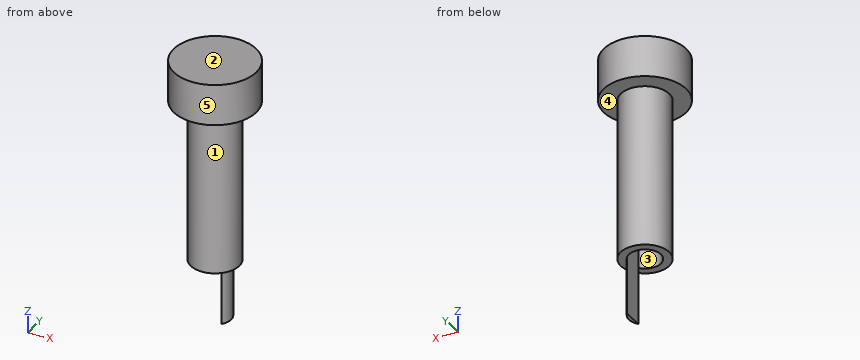
from build123d import *

# Parameters (mm, degrees)
BOSS_EXTRUDE1_DEPTH = 9.906
SKETCH6_R           = 1.975
BOSS_EXTRUDE2_DEPTH = 17.272
SKETCH7_R           = 2.99147738
BOSS_EXTRUDE3_DEPTH = 20.066
CUT_EXTRUDE1_DEPTH  = 20.066
SKETCH9_R           = 5.08
BOSS_EXTRUDE4_DEPTH = 5.08


with BuildPart() as part:
    # Sketch5 → Boss-Extrude1 (new body)
    with BuildSketch(Plane.XY):
        with BuildLine():
            Line((1.525, 0), (1.525, 1.25499004))
            ThreePointArc((1.525, 1.25499004), (1.975, 0), (1.525, -1.25499004))
            Line((1.525, -1.25499004), (1.525, 0))
        make_face()
    extrude(amount=BOSS_EXTRUDE1_DEPTH)

    # Sketch6 → Boss-Extrude2 (add)
    with BuildSketch(Plane.XY.offset(9.906)):
        Circle(SKETCH6_R)
    extrude(amount=BOSS_EXTRUDE2_DEPTH)

    # Sketch7 → Boss-Extrude3 (add)
    with BuildSketch(Plane.XY.offset(27.178)):
        Circle(SKETCH7_R)
    extrude(amount=-BOSS_EXTRUDE3_DEPTH)

    # Sketch8 → Cut-Extrude1 (cut)
    with BuildSketch(Plane.XY):
        with BuildLine():
            Line((1.525, 1.25499004), (1.525, 0))
            Line((1.525, 0), (1.525, -1.25499004))
            ThreePointArc((1.525, -1.25499004), (-1.975, 0), (1.525, 1.25499004))
        make_face()
    extrude(amount=CUT_EXTRUDE1_DEPTH, mode=Mode.SUBTRACT)

    # Sketch9 → Boss-Extrude4 (add)
    with BuildSketch(Plane.XY.offset(27.178)):
        Circle(SKETCH9_R)
    extrude(amount=BOSS_EXTRUDE4_DEPTH)


solid = part.part
Geometry check sheet. Reference: the model listing, model coordinates, mm. Face numbers are marked on the shaded views. A direction names the side the tool comes from. Coordinates: 2 decimals unless noted, no trailing zeros. Write each loop counter-clockwise with the first axis right and the second up, starting at its lowest first coordinate (ties: lowest second). Pieces come first, ordered by that corner, then holes. Notation, with made-up numbers: (-33.5, -6.75) -> (8.5, -6.75) arc R21 cw to (8.5, 23.25) -> close; hole circle Ø7 at (46, 62.5). An arc over 180 degrees is marked (long way). One line per question, with ' | ' between items.
1. Set-up check for the marked faces 4 and 5: record each of +Z, -Z, +X, -X, +Y, -Y from which the full face is reachable in a straight line by a thin tool's end or side.
Answers:
face 4: -Z | face 5: +Z, -Z
2. Draft check along Y on the marked faces 1, 2 and 3. Enter one of: +Y half, -Y half, draft (parallel to the pull), parting line (faces both ways), or undercut.
Answers:
face 1: parting line | face 2: draft | face 3: undercut
3. Cross-section at A-A on x = 0. Record the cut outline in (y, z) (3 decimals).
Answers:
outline: (-5.08, 27.178) -> (-2.991, 27.178) -> (-2.991, 7.112) -> (-1.975, 7.112) -> (-1.975, 20.066) -> (1.975, 20.066) -> (1.975, 7.112) -> (2.991, 7.112) -> (2.991, 27.178) -> (5.08, 27.178) -> (5.08, 32.258) -> (-5.08, 32.258) -> close
4. Cross-section at B-B on y = 0. Record the cut outline in (x, z) (3 decimals), and give its area (3 significant figures).
Answers:
outline: (-5.08, 27.178) -> (-2.991, 27.178) -> (-2.991, 7.112) -> (-1.975, 7.112) -> (-1.975, 20.066) -> (1.525, 20.066) -> (1.525, 0) -> (1.975, 0) -> (1.975, 7.112) -> (2.991, 7.112) -> (2.991, 27.178) -> (5.08, 27.178) -> (5.08, 32.258) -> (-5.08, 32.258) -> close | area: 130 mm²
5. Cross-section at C-C on z = 12.5. Record the cut outline in (x, y) (3 decimals).
Answers:
outline: circle Ø5.983 at (0, 0); hole (1.525, -1.255) -> (1.525, 1.255) arc R1.975 ccw (long way) to start
6. Depth check by flat-ended pin: pin 1 Ø3 at (y, z) = (3, 17) entering from +X; pin 2 Ø2 at (y, z) = (-2.5, 5.5) entering from -X; pin 3 Ø6 at (y, z) = (0.5, 10) entering from -X; pin 4 Ø1.5 at (y, z) = (1, 19.5) entering from +X. Enter the tip coordinate at first touch or a pass-through.
Answers:
pin 1: stops at x = 2.59 | pin 2: passes through | pin 3: stops at x = -2.99 | pin 4: stops at x = 2.98
7. Cross-section at D-D on z = 23. Record the cut outline in (x, y).
Answers:
outline: circle Ø5.98 at (0, 0)
8. Thickness scan on probe 1 along Y at (x, z) = (0, 14) (3 decimals); probe 2 along Z at (x, y) = (-3, 0.5); probe 3 along X at (y, z) = (-0.5, 13) (3 decimals). Record the ranges inside material, lowest first. Write a range as from..to.
Answers:
probe 1: y = -2.991..-1.975, 1.975..2.991 | probe 2: z = 27.18..32.26 | probe 3: x = -2.949..-1.911, 1.525..2.949
